Can you work these out from the model? Positions are in its coordinate system, mm. A direction names the side the tool comes from. Coordinates: 2 decimals unless noted, no trailing zeros. Write each loop counter-clockwise with the first axis right and the second up, starting at its lowest first coordinate (ties: lowest second). Pieces come first, ordered by that corner, then holes. Notation, with made-up numbers: (21.5, 28) - (46.5, 28) arc R21 ccw to (46.5, 42) - close; hole circle Ø4 at (75.25, 36). An arc over 180 degrees is marked (long way). Use one line per item in the form item = value. Start each with the question number.
(1) On a 3-axis mill with a long thin cutter (end or side, diameter ignored), from which of +Z, -Z, +X, -X, +Y, -Y can I reach the whole of each face in a straight line? I mean faces 4 (the face through (9.027, 13.114, -0.195)), 5 (the face through (9.86, 2.028, 4.24)), 6 (the face through (12.163, -1.726, 0.215)), 7 (the face through (10, 1, 5.2)). Say none if no direction works.
(2) For pin 1 Ø1.5 at (x, z) = (12.5, 0) entering from +Y; pin 2 Ø1 at (x, y) = (14, 4) entering from +Z; pin 3 Ø1 at (x, z) = (13, 2.5) entering from +Y, each with a flat end and sliding along its axis, tell me the tip position at first contact or that it passes through.
(3) Thinking about a two-plate mould opening in X: for faces 1 (the face through (0, 7, 0)), 2 (the face through (9.86, 12.499, 2.514)), 3 (the face through (18, 12.1, 0)), which applies, pulls with the +X half, pulls with the -X half, needs draft (parallel to the pull), parting line crosses it, or undercut?
(4) If we section it at D-D on x = 3.75: Please give me the cut outline in (y, z).
(5) If we section it at C-C on y = -1: Please give me the cut outline in (x, z), then the cut area to 3 significant figures.
(6) If we section it at A-A on x = 10.75: Please give me the cut outline in (y, z).
(7) If I drill on probe 1 along X at (y, z) = (13.7, 0); probe 2 along Y at (x, z) = (6.75, -0.75); probe 3 along X at (y, z) = (-1.75, -0.25), over which ranges is the centre line in solid material (lowest first)? Write a range as from..to.
(8) If we section it at B-B on y = 13.25: Please give me the cut outline in (x, z), then the cut area to 3 significant figures.
```python
from build123d import *

# Parameters (mm, degrees)
EXTRUDE_1_DEPTH     = 20
SKETCH_2_R          = 1.5
CUT_EXTRUDE_1_DEPTH = 2
SKETCH_3_R          = 0.4
EXTRUDE_2_DEPTH     = 3.5


with BuildPart() as part:
    # 草图1 → 凸台-拉伸1 (new body)
    with BuildSketch(Plane(origin=(0, 0, 0), x_dir=(0, 0, -1), z_dir=(1, 0, 0))):
        Polygon((0, 0), (5, 0), (5, 6.798949449), (1.592861235, 14.1), (-1.592861235, 14.1), (-3.462246636, 10.852770352), (-5.2, 10.041823104), (-5.2, 6.798949449), (-3.305827132, 5.708500208), (-3.305827132, 2.534594125), (-5.2, 1.506142854), (-5.2, 0), align=None)
    extrude(amount=EXTRUDE_1_DEPTH)

    # 草图2 → 切除-拉伸1 (cut)
    with BuildSketch(Plane(origin=(0, 14.1, 0), x_dir=(1, 0, 0), z_dir=(0, 1, 0))):
        with Locations(Location((2.54, 0, 0), (0, 0, 270))):
            Circle(SKETCH_2_R)
        with Locations(Location((7.54, 0, 0), (0, 0, 270))):
            Circle(SKETCH_2_R)
        with Locations(Location((12.54, 0, 0), (0, 0, 270))):
            Circle(SKETCH_2_R)
        with Locations(Location((17.54, 0, 0), (0, 0, 270))):
            Circle(SKETCH_2_R)
    extrude(amount=-CUT_EXTRUDE_1_DEPTH, mode=Mode.SUBTRACT)

    # 草图3 → 凸台-拉伸2 (add)
    with BuildSketch(Plane.XZ):
        with Locations(Location((2.5, 0, 0), (0, 0, 90))):
            Circle(SKETCH_3_R)
        with Locations(Location((7.5, 0, 0), (0, 0, 90))):
            Circle(SKETCH_3_R)
        with Locations(Location((12.5, 0, 0), (0, 0, 90))):
            Circle(SKETCH_3_R)
        with Locations(Location((17.5, 0, 0), (0, 0, 90))):
            Circle(SKETCH_3_R)
    extrude(amount=EXTRUDE_2_DEPTH)


solid = part.part
```
Reported:
q1.face_4 = +Y
q1.face_5 = +Z, +X, -X
q1.face_6 = -Y
q1.face_7 = +Z, +X, -X, +Y, -Y
q2.pin_1 = 12.1
q2.pin_2 = 3.31
q2.pin_3 = 13.39
q3.face_1 = pulls with the -X half
q3.face_2 = needs draft
q3.face_3 = undercut
q4.outline = (0, -5) - (6.8, -5) - (14.1, -1.59) - (14.1, -0.89) - (12.1, -0.89) - (12.1, 0.89) - (14.1, 0.89) - (14.1, 1.59) - (10.85, 3.46) - (10.04, 5.2) - (6.8, 5.2) - (5.71, 3.31) - (2.53, 3.31) - (1.51, 5.2) - (0, 5.2) - close
q5.outline = circle Ø0.8 at (2.5, 0); circle Ø0.8 at (7.5, 0); circle Ø0.8 at (12.5, 0); circle Ø0.8 at (17.5, 0)
q5.area = 2.01 mm2
q6.outline = (0, -5) - (6.8, -5) - (14.1, -1.59) - (14.1, 1.59) - (10.85, 3.46) - (10.04, 5.2) - (6.8, 5.2) - (5.71, 3.31) - (2.53, 3.31) - (1.51, 5.2) - (0, 5.2) - close
q7.probe_1 = 0..1.04, 4.04..6.04, 9.04..11.04, 14.04..16.04, 19.04..20
q7.probe_2 = 0..12.1
q7.probe_3 = 2.19..2.81, 7.19..7.81, 12.19..12.81, 17.19..17.81
q8.outline = (0, -1.99) - (20, -1.99) - (20, 2.08) - (0, 2.08) - close; hole circle Ø3 at (2.54, 0); hole circle Ø3 at (7.54, 0); hole circle Ø3 at (12.54, 0); hole circle Ø3 at (17.54, 0)
q8.area = 53.2 mm2
